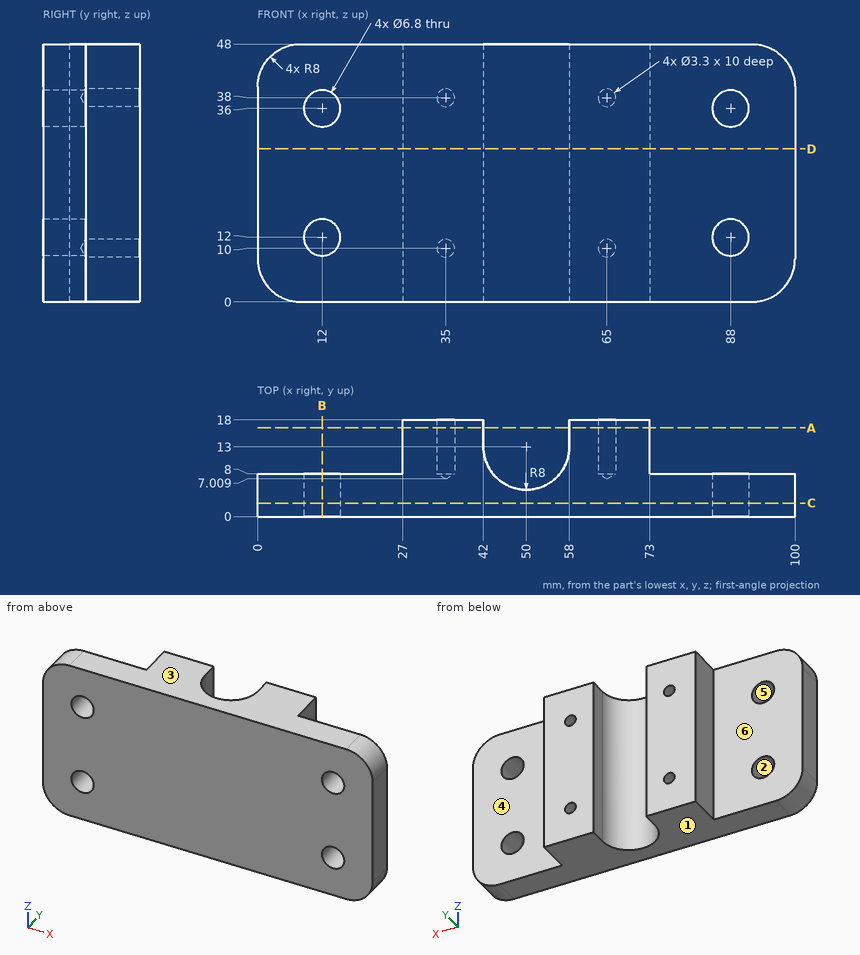
For this review, use the dimensioned drawing (mm, ordinates from the lowest corner) and the shaded views. A direction names the side the tool comes from. Give positions to 0.01 mm unless a question says otherwise; leave off trailing zeros. Order: outer loops, then holes, each group sorted by start corner. A loop starts at its lowest first (then second) coordinate and runs counter-clockwise, first axis right, second up. Notation, with made-up numbers: (78, -4) - (94, -4) arc R20 ccw to (94, 32) - close; hole circle Ø7 at (-4, 36). An arc over 180 degrees is marked (long way). Use a Markdown table: item, result. Add a question column.
(1) Mouldability with a two-part tool opening along Z and no side actions: class the marked faces 1, 2 and 3 as +Z half, -Z half, draft (parallel to the pull), parting line (faces both ways), or undercut.
(2) Clearance check with flat-ended pins moving along their axes: P1, Ø2, axis at x = 65, z = 10, coming from the +Y side; P2, Ø1.5, axis at y = 15, z = 28, coming from the +X side; P3, Ø13.5, axis at x = 92, z = 20, coming from the +Y side. State where each tip first meets the part, or that it passes through.
(3) Add section D-D on z = 28.5. Give the boundary of the cut face in (x, y).
(4) Machinability: for the marked faces 4, 5 and 6, which of the approach directions +Z, -Z, +X, -X, +Y, -Y give a long, thin tool a straight path to every point of the face, cutting with its end or side? Answer none if there is none.
(5) Add section C-C on y = 2.5. Give the boundary of the cut face in (x, z), then the cut area to 3 significant figures.
(6) Wall thickness on probe 1 along Z at (x, y) = (35, 15.5); probe 2 along Z at (x, y) = (88, 1.25); probe 3 along X at (y, z) = (14.25, 42): over which ranges is each line inside the solid? List them lowest first. Write a range as [from, to].
(7) Add section A-A on y = 16.5. Give the boundary of the cut face in (x, z), then the cut area to 3 significant figures.
(8) Add section B-B on x = 12. Give the boundary of the cut face in (y, z).
Report:
| question | item | result |
|---|---|---|
| 1 | face 1 | -Z half |
| 1 | face 2 | undercut |
| 1 | face 3 | +Z half |
| 2 | P1 | stops at y = 7.61 |
| 2 | P2 | stops at x = 73 |
| 2 | P3 | stops at y = 8 |
| 3 | outline | (0, 0) - (100, 0) - (100, 8) - (73, 8) - (73, 18) - (58, 18) - (58, 13) arc R8 cw to (42, 13) - (42, 18) - (27, 18) - (27, 8) - (0, 8) - close |
| 4 | face 4 | +Z, -Z, +X, +Y |
| 4 | face 5 | +Y, -Y |
| 4 | face 6 | +Z, -Z, -X, +Y |
| 5 | outline | (0, 8) arc R8 ccw to (8, 0) - (92, 0) arc R8 ccw to (100, 8) - (100, 40) arc R8 ccw to (92, 48) - (8, 48) arc R8 ccw to (0, 40) - close; hole circle Ø6.8 at (12, 12); hole circle Ø6.8 at (12, 36); hole circle Ø6.8 at (88, 12); hole circle Ø6.8 at (88, 36) |
| 5 | area | 4,600 mm² |
| 6 | probe 1 | z = [0, 8.35], [11.65, 36.35], [39.65, 48] |
| 6 | probe 2 | z = [0, 8.6], [15.4, 32.6], [39.4, 48] |
| 6 | probe 3 | x = [27, 42], [58, 73] |
| 7 | outline | (27, 0) - (42, 0) - (42, 48) - (27, 48) - close; (58, 0) - (73, 0) - (73, 48) - (58, 48) - close; hole circle Ø3.3 at (35, 10); hole circle Ø3.3 at (35, 38); hole circle Ø3.3 at (65, 10); hole circle Ø3.3 at (65, 38) |
| 7 | area | 1,410 mm² |
| 8 | outline | (0, 0) - (8, 0) - (8, 8.6) - (0, 8.6) - close; (0, 15.4) - (8, 15.4) - (8, 32.6) - (0, 32.6) - close; (0, 39.4) - (8, 39.4) - (8, 48) - (0, 48) - close |
